```python
from build123d import *

# Parameters (mm, degrees)
F1_DEPTH = 10.16
F3_DEPTH = 7.62
F5_DEPTH = 25.4


with BuildPart() as f1:
    # F0 (on Front) → F1 (new body)
    with BuildSketch(Plane.XZ):
        with BuildLine():
            Line((55.499, 31.877), (-55.499, 31.877))
            ThreePointArc((-55.499, 31.877), (-61.785179, 29.273179), (-64.389, 22.987))
            Line((-64.389, 22.987), (-64.389, -22.987))
            ThreePointArc((-64.389, -22.987), (-61.785179, -29.273179), (-55.499, -31.877))
            Line((-55.499, -31.877), (55.499, -31.877))
            ThreePointArc((55.499, -31.877), (61.785179, -29.273179), (64.389, -22.987))
            Line((64.389, -22.987), (64.389, 22.987))
            ThreePointArc((64.389, 22.987), (61.785179, 29.273179), (55.499, 31.877))
        make_face()
    extrude(amount=F1_DEPTH)

    # F2 (on face) → F3 (cut)
    with BuildSketch(Plane.XZ.offset(10.16)):
        with BuildLine():
            Line((55.499, 29.337), (-55.499, 29.337))
            ThreePointArc((-55.499, 29.337), (-59.989128, 27.477128), (-61.849, 22.987))
            Line((-61.849, 22.987), (-61.849, -22.987))
            ThreePointArc((-61.849, -22.987), (-59.989128, -27.477128), (-55.499, -29.337))
            Line((-55.499, -29.337), (55.499, -29.337))
            ThreePointArc((55.499, -29.337), (59.989128, -27.477128), (61.849, -22.987))
            Line((61.849, -22.987), (61.849, 22.987))
            ThreePointArc((61.849, 22.987), (59.989128, 27.477128), (55.499, 29.337))
        make_face()
    extrude(amount=-F3_DEPTH, mode=Mode.SUBTRACT)

    # F4 (on face) → F5 (cut)
    with BuildSketch(Plane(origin=(0, 0, 0), x_dir=(-1, 0, 0), z_dir=(0, 1, 0))):
        with BuildLine():
            ThreePointArc((-61.394893, -21.146874), (-59.906995, -24.738976), (-56.314893, -26.226874))
            Line((-56.314893, -26.226874), (-56.235034, -26.226874))
            ThreePointArc((-56.235034, -26.226874), (-52.642932, -24.738976), (-51.155034, -21.146874))
            Line((-51.155034, -21.146874), (-51.155034, -12.330383))
            ThreePointArc((-51.155034, -12.330383), (-52.642932, -8.738281), (-56.235034, -7.250383))
            Line((-56.235034, -7.250383), (-56.314893, -7.250383))
            ThreePointArc((-56.314893, -7.250383), (-59.906995, -8.738281), (-61.394893, -12.330383))
            Line((-61.394893, -12.330383), (-61.394893, -21.146874))
        make_face()
    extrude(amount=-F5_DEPTH, mode=Mode.SUBTRACT)


solid = f1.part
```
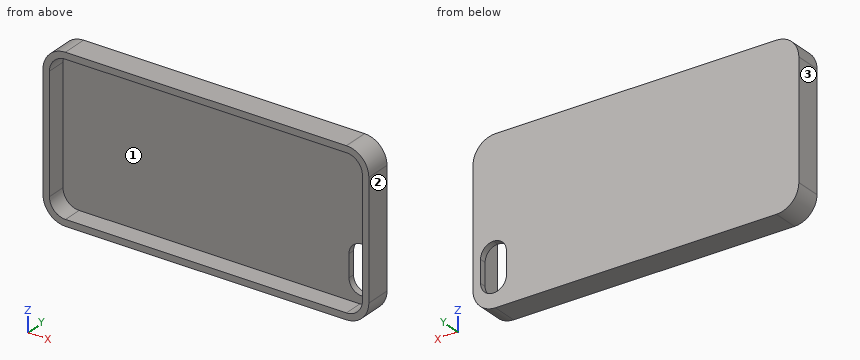
Could you check a few things on this model? Use its own coordinates, in mm. Face numbers are marked on the shaded views. Give positions to 0.01 mm unless a question says otherwise; leave off trailing zeros. Write each loop counter-clockwise with the first axis right and the second up, starting at its lowest first coordinate (ties: lowest second). Pieces come first, ordered by that corner, then holes. Notation, with made-up numbers: (14, 32.25) -> (20, 32.25) arc R20 ccw to (20, 56.25) -> close; hole circle Ø10 at (81, 12.25). An arc over 180 degrees is marked (long way). Write each question's results on one line, items separated by ' | '.
1. I want a section at B-B, the plane y = -8. Write out the boundary of the cut face in (x, z), then the cut area to 3 significant figures.
Check sheet entries:
outline: (-64.39, -22.99) arc R8.89 ccw to (-55.5, -31.88) -> (55.5, -31.88) arc R8.89 ccw to (64.39, -22.99) -> (64.39, 22.99) arc R8.89 ccw to (55.5, 31.88) -> (-55.5, 31.88) arc R8.89 ccw to (-64.39, 22.99) -> close; hole (-61.85, -22.99) arc R6.35 ccw to (-55.5, -29.34) -> (55.5, -29.34) arc R6.35 ccw to (61.85, -22.99) -> (61.85, 22.99) arc R6.35 ccw to (55.5, 29.34) -> (-55.5, 29.34) arc R6.35 ccw to (-61.85, 22.99) -> close | area: 919 mm²
2. I want a section at C-C, the plane x = 24.5. Write out the boundary of the cut face in (y, z).
Check sheet entries:
outline: (-10.16, -31.88) -> (0, -31.88) -> (0, 31.88) -> (-10.16, 31.88) -> (-10.16, 29.34) -> (-2.54, 29.34) -> (-2.54, -29.34) -> (-10.16, -29.34) -> close
3. I need wall thicknesses on L1, parallel to Z at x = -29, y = -8; L2, parallel to X at y = -7.75, z = 19.5; L3, parallel to X at y = -1, z = -25. Which ranges of each line are inside material? Lowest first, please.
Check sheet entries:
L1: z = -31.88 to -29.34, 29.34 to 31.88 | L2: x = -64.39 to -61.85, 61.85 to 64.39 | L3: x = -64.16 to 52.92, 59.63 to 64.16
4. I want a section at D-D, the plane z = -6. Write out the boundary of the cut face in (x, y), then the cut area to 3 significant figures.
Check sheet entries:
outline: (-64.39, -10.16) -> (-61.85, -10.16) -> (-61.85, -2.54) -> (61.85, -2.54) -> (61.85, -10.16) -> (64.39, -10.16) -> (64.39, 0) -> (-64.39, 0) -> close | area: 366 mm²
5. If we mould it in two halves opening along X, with no side actions, what happens to the marked faces 1, 2 and 3? For each: released by +X, released by -X, zero draft, split by the parting line, or undercut.
Check sheet entries:
face 1: undercut | face 2: released by +X | face 3: released by -X
6. I want a section at A-A, the plane z = -18. Write out the boundary of the cut face in (x, y).
Check sheet entries:
outline: (-64.39, -10.16) -> (-61.85, -10.16) -> (-61.85, -2.54) -> (51.16, -2.54) -> (51.16, 0) -> (-64.39, 0) -> close; (61.39, -2.54) -> (61.85, -2.54) -> (61.85, -10.16) -> (64.39, -10.16) -> (64.39, 0) -> (61.39, 0) -> close
7. Will this pin go through, and if not, where does the flat tip stop? pin 1 Ø4 at (x, z) = (-26.5, 22) entering from -Y.
Check sheet entries:
pin 1: stops at y = -2.54
